Verification items for the finished model (mm, model axes). Coordinates: 2 decimals unless noted, no trailing zeros. Order: outer loops, then holes, each group sorted by start corner. A loop starts at its lowest first (then second) coordinate and runs counter-clockwise, first axis right, second up. Notation, with made-up numbers: M -37,31 L -23,31 A22 ccw -23,57 Z; hole C 65,-11 d3. An arc over 180 degrees is marked long. Write item = value, one per line.
```python
from build123d import *

# Parameters (mm, degrees)
F0_W            = 95
F0_H            = 95
F1_DEPTH        = 5.5
F2_R            = 20
F3_R            = 11
F4_DEPTH        = 5.5
F6_D            = 3.5
F6_CSINK_D      = 8.5
F6_CSINK_ANGLE  = 90
F8_D            = 3.5
F8_CSINK_D      = 8.5
F8_CSINK_ANGLE  = 90
F10_D           = 3.5
F10_CSINK_D     = 8.5
F10_CSINK_ANGLE = 90


with BuildPart() as f1:
    # F0 (on Top) → F1 (new body)
    with BuildSketch(Plane.XY):
        Rectangle(F0_W, F0_H)
    extrude(amount=F1_DEPTH)

    # F2
    f2_edges = [f1.edges().sort_by_distance(p)[0] for p in [
        (47.5, -47.5, 2.75),
        (47.5, 47.5, 2.75),
        (-47.5, 47.5, 2.75),
        (-47.5, -47.5, 2.75),
    ]]
    fillet(f2_edges, radius=F2_R)

    # F3 (on face) → F4 (cut)
    with BuildSketch(Plane.XY.offset(5.5)):
        Circle(F3_R)
    extrude(amount=-F4_DEPTH, mode=Mode.SUBTRACT)

    # F6 (through all)
    with Locations(Plane(origin=(0, 0, 0), x_dir=(1, 0, 0), z_dir=(0, 0, -1))):
        with Locations((0, -40), (0, 40), (40, 0), (-40, 0)):
            CounterSinkHole(F6_D / 2, F6_CSINK_D / 2, counter_sink_angle=F6_CSINK_ANGLE)

    # F8 (through all)
    with Locations(Plane(origin=(0, 0, 0), x_dir=(1, 0, 0), z_dir=(0, 0, -1))):
        with Locations((-13.188658, 40), (12.085494, 40), (40, 10.745424), (40, -12.022199), (12.085494, -40), (-13.188658, -40), (-40, -10.351182), (-40, 10.745424)):
            CounterSinkHole(F8_D / 2, F8_CSINK_D / 2, counter_sink_angle=F8_CSINK_ANGLE)

    # F10 (through all)
    with Locations(Plane(origin=(0, 0, 0), x_dir=(1, 0, 0), z_dir=(0, 0, -1))):
        with Locations((-22.5, 22.5), (22.5, 22.5), (22.5, -22.5), (-22.5, -22.5)):
            CounterSinkHole(F10_D / 2, F10_CSINK_D / 2, counter_sink_angle=F10_CSINK_ANGLE)


solid = f1.part
```
Item 1: Sectioned sample at B-B, the plane y = 0. Enter the section's corners in (x, z), then the cut area to 4 significant figures.
Report:
outline = M -47.5,0 L -44.25,0 L -41.75,2.5 L -41.75,5.5 L -47.5,5.5 Z; M -38.25,2.5 L -35.75,0 L -11,0 L -11,5.5 L -38.25,5.5 Z; M 11,0 L 35.75,0 L 38.25,2.5 L 38.25,5.5 L 11,5.5 Z; M 41.75,2.5 L 44.25,0 L 47.5,0 L 47.5,5.5 L 41.75,5.5 Z
area = 350.5 mm^2
Item 2: Scan lines: L1, parallel to X at y = -22.5, z = 4; L2, parallel to Y at x = -39, z = 2.3. Record each from-to range of solid material in increasing order. Write a range as from..to.
Report:
L1 = -47.5..-24.25, -20.75..20.75, 24.25..47.5
L2 = -43.86..-12.42, -9.07..-1.67, 1.67..8.68, 12.03..43.86
Item 3: Sectioned sample at A-A, the plane x = -22.5. Enter the section's corners in (y, z), then the cut area to 4 significant figures.
Report:
outline = M -47.5,0 L -26.75,0 L -24.25,2.5 L -24.25,5.5 L -47.5,5.5 Z; M -20.75,2.5 L -18.25,0 L 18.25,0 L 20.75,2.5 L 20.75,5.5 L -20.75,5.5 Z; M 24.25,2.5 L 26.75,0 L 47.5,0 L 47.5,5.5 L 24.25,5.5 Z
area = 471.5 mm^2
Item 4: Release check for a two-part mould opening along Y. For faces 1 (the cylindrical face through (-14, 41.55, 4.02)), 2 (the cylindrical face through (41.486, -41.797, 2.788)), 3 (the flat face through (-0.7, 11.2, 5.5)) record: pulls with the +Y half, pulls with the -Y half, needs draft (parallel to the pull), parting line crosses it, or undercut.
Report:
face_1 = undercut
face_2 = pulls with the -Y half
face_3 = needs draft
Item 5: Gauge pin test, flat ends, axial feed: pin 1 (4.5 mm diameter, centred on x = 0, y = -40, fed in from -Z); pin 2 (5.5 mm diameter, centred on x = 22.5, y = -22.5, fed in from -Z). Record the tip position at first contact, or that the pin passes through.
Report:
pin_1 = 2
pin_2 = 1.5
Item 6: Sectioned sample at D-D, the plane z = 4.05. Give the number of separate pieces and of enclosed holes in the cut face, then the cut area to 3 significant figures.
Report:
separate_pieces = 1
enclosed_holes = 17
area = 8,150 mm^2
